```python
from build123d import *

# Parameters (mm, degrees)
BOSS_EXTRUDE1_DEPTH = 25.4
SKETCH2_W           = 7.790615149
SKETCH2_H           = 25.4
BOSS_EXTRUDE2_DEPTH = 3.048
SKETCH3_R           = 7.790615149
BOSS_EXTRUDE3_DEPTH = 25.4


with BuildPart() as part:
    # Sketch1 → Boss-Extrude1 (new body)
    with BuildSketch(Plane.XY):
        Polygon((-38.1, 0), (38.1, 0), (38.1, 10.1092), (12.442422535, 10.1092), (12.442422535, 6.0706), (36.322, 6.0706), (36.322, 2.032), (-36.322, 2.032), (-36.322, 6.0706), (-12.442422535, 6.0706), (-12.442422535, 10.1092), (-38.1, 10.1092), align=None)
    extrude(amount=-BOSS_EXTRUDE1_DEPTH)

    # Sketch2 → Boss-Extrude2 (add)
    with BuildSketch(Plane.XY):
        with Locations((-3.895307575, -12.7)):
            Rectangle(SKETCH2_W, SKETCH2_H)
        with Locations((3.895307575, -12.7)):
            Rectangle(SKETCH2_W, SKETCH2_H)
    extrude(amount=-BOSS_EXTRUDE2_DEPTH)

    # Sketch3 → Boss-Extrude3 (add)
    with BuildSketch(Plane(origin=(0, 0, 0), x_dir=(-1, 0, 0), z_dir=(0, 0, -1))):
        with Locations((0, -25.4)):
            Circle(SKETCH3_R)
    extrude(amount=BOSS_EXTRUDE3_DEPTH)


solid = part.part
```
Can you work these out from the model? Positions are in its coordinate system, mm. A direction names the side the tool comes from. Give positions to 0.01 mm unless a question says otherwise; leave off trailing zeros. Loops run counter-clockwise (first coordinate to the right, second up) from the corner with the lowest first, then second, coordinate; pieces in that order, holes last. Notation, with made-up numbers: M 60,-27 L 114,-27 A17 cw 114,3 Z; hole C 79,-20.5 d1. An arc over 180 degrees is marked long. Use CSV: the item, a comma, the result in double quotes. Start each with the question number.
1. Imagine slicing it at A-A, the plane y = 4.5. Write out the boundary of the cut face in (x, z).
2. For P1, Ø2, axis at y = -24, z = -11.5, coming from the +X side; P2, Ø7, axis at x = -23.5, z = -10, coming from the -Y side; P3, Ø7.5, axis at x = -7.5, z = -18, coming from the +Y side, each with a flat end and sliding along its axis, tell me the tip position at first contact or that it passes through.
3. If I drill on L1, parallel to Y at x = -34, z = -22.5; L2, parallel to Y at x = -11, z = -5.75; L3, parallel to X at y = 4, z = -5.75, over which ranges is the centre line in solid material (lowest first)?
4. Imagine slicing it at B-B, the plane z = -9.5. Write out the boundary of the cut face in (x, y).
5. On a 3-axis mill with a long thin cutter (end or side, diameter ignored), from which of +Z, -Z, +X, -X, +Y, -Y can I reach the whole of each face in a straight line? I mean faces 1 (the face through (1.689, -33.005, -12.522)), 2 (the face through (24, 6.071, -13)), 3 (the face through (7.791, -13, -2)), 4 (the face through (-12.442, 8, -13)), 5 (the face through (-7.791, -13, -2)). Say none if no direction works.
6. If we mould it in two halves opening along Y, with no side actions, what happens to faces 6 (the face through (25, 10.109, -13)), 7 (the face through (36.322, 4, -13)), 8 (the face through (38.1, 5, -13))? For each: released by +Y, released by -Y, zero draft, split by the parting line, or undercut.
7. Imagine slicing it at C-C, the plane x = 0. Write out the boundary of the cut face in (y, z), plus the area to 3 significant figures.
8. Imagine slicing it at D-D, the plane y = -19. Write out the boundary of the cut face in (x, z), plus the area to 3 significant figures.
Response values:
1,outline,"M -38.1,-25.4 L -36.32,-25.4 L -36.32,0 L -38.1,0 Z; M 36.32,-25.4 L 38.1,-25.4 L 38.1,0 L 36.32,0 Z"
2,P1,"x = 7.78"
2,P2,"y = 0"
2,P3,"y = 2.03"
3,L1,"0 to 2.03, 6.07 to 10.11"
3,L2,"0 to 2.03"
3,L3,"-38.1 to -36.32, 36.32 to 38.1"
4,outline,"M -38.1,0 L 38.1,0 L 38.1,10.11 L 12.44,10.11 L 12.44,6.07 L 36.32,6.07 L 36.32,2.03 L -36.32,2.03 L -36.32,6.07 L -12.44,6.07 L -12.44,10.11 L -38.1,10.11 Z; C 0,-25.4 d15.58"
5,face 1,"-Z"
5,face 2,"+Z, -Z"
5,face 3,"+Z, -Z, +X, -Y"
5,face 4,"+Z, -Z, +Y"
5,face 5,"+Z, -Z, -X, -Y"
6,face 6,"released by +Y"
6,face 7,"undercut"
6,face 8,"zero draft"
7,outline,"M -33.19,-25.4 L -17.61,-25.4 L -17.61,-3.05 L 0,-3.05 L 0,-25.4 L 2.03,-25.4 L 2.03,0 L -33.19,0 Z"
7,area,"501 mm^2"
8,outline,"M -7.79,-3.05 L -4.44,-3.05 L -4.44,-25.4 L 4.44,-25.4 L 4.44,-3.05 L 7.79,-3.05 L 7.79,0 L -7.79,0 Z"
8,area,"246 mm^2"
